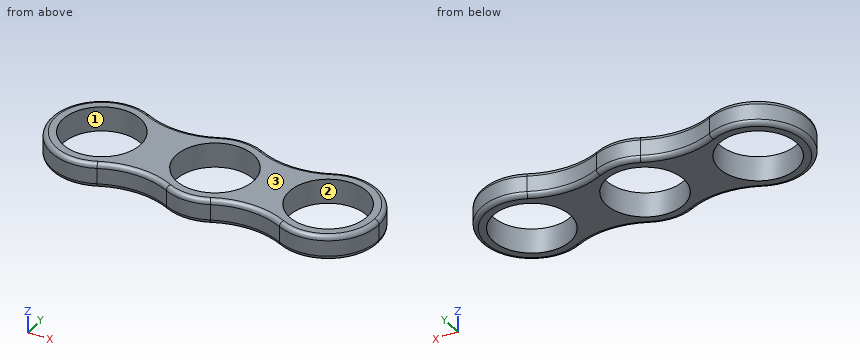
```python
from build123d import *

# Parameters (mm, degrees)
F0_R     = 11
F1_DEPTH = 7
F2_R     = 1.27


with BuildPart() as f1:
    # F0 (on Top) → F1 (new body)
    with BuildSketch(Plane.XY):
        with BuildLine():
            ThreePointArc((6.1706337368, -12.8862692637), (12.0891601396, -7.6147792724), (14.2875, 0))
            ThreePointArc((14.2875, 0), (12.0891601396, 7.6147792724), (6.1706337368, 12.8862692637))
            ThreePointArc((6.1706337368, 12.8862692637), (0, 14.2875), (-6.1706337368, 12.8862692637))
            ThreePointArc((-6.1706337368, 12.8862692637), (-14.2875, 0), (-6.1706337368, -12.8862692637))
            ThreePointArc((-6.1706337368, -12.8862692637), (0, -14.2875), (6.1706337368, -12.8862692637))
        make_face()
        Circle(F0_R, mode=Mode.SUBTRACT)
        with BuildLine():
            ThreePointArc((6.1706337368, 12.8862692637), (12.0891601396, 7.6147792724), (14.2875, 0))
            ThreePointArc((14.2875, 0), (12.0891601396, -7.6147792724), (6.1706337368, -12.8862692637))
            ThreePointArc((6.1706337368, -12.8862692637), (15.875, -10.6825966971), (25.5793662632, -12.8862692637))
            ThreePointArc((25.5793662632, -12.8862692637), (17.4625, 0), (25.5793662632, 12.8862692637))
            ThreePointArc((25.5793662632, 12.8862692637), (15.875, 10.6825966971), (6.1706337368, 12.8862692637))
        make_face()
        with BuildLine():
            ThreePointArc((-6.1706337368, -12.8862692637), (-14.2875, 0), (-6.1706337368, 12.8862692637))
            ThreePointArc((-6.1706337368, 12.8862692637), (-15.875, 10.6825966971), (-25.5793662632, 12.8862692637))
            ThreePointArc((-25.5793662632, 12.8862692637), (-19.6608398604, 7.6147792724), (-17.4625, 0))
            ThreePointArc((-17.4625, 0), (-19.6608398604, -7.6147792724), (-25.5793662632, -12.8862692637))
            ThreePointArc((-25.5793662632, -12.8862692637), (-15.875, -10.6825966971), (-6.1706337368, -12.8862692637))
        make_face()
        with BuildLine():
            ThreePointArc((46.0375, 0), (39.3647792724, 12.0891601396), (25.5793662632, 12.8862692637))
            ThreePointArc((25.5793662632, 12.8862692637), (17.4625, 0), (25.5793662632, -12.8862692637))
            ThreePointArc((25.5793662632, -12.8862692637), (39.3647792724, -12.0891601396), (46.0375, 0))
        make_face()
        with Locations((31.75, 0)):
            Circle(F0_R, mode=Mode.SUBTRACT)
        with BuildLine():
            ThreePointArc((-17.4625, 0), (-19.6608398604, 7.6147792724), (-25.5793662632, 12.8862692637))
            ThreePointArc((-25.5793662632, 12.8862692637), (-46.0375, 0), (-25.5793662632, -12.8862692637))
            ThreePointArc((-25.5793662632, -12.8862692637), (-19.6608398604, -7.6147792724), (-17.4625, 0))
        make_face()
        with Locations((-31.75, 0)):
            Circle(F0_R, mode=Mode.SUBTRACT)
    extrude(amount=F1_DEPTH)

    # F2
    f2_edges = [f1.edges().sort_by_distance(p)[0] for p in [
        (-46.0375, 0, 7),
        (0, 14.2875, 0),
    ]]
    fillet(f2_edges, radius=F2_R)


solid = f1.part
```
Work out the finished part from the listing and answer in its coordinate system (mm). Face numbers are marked on the shaded views. Coordinates: 2 decimals unless noted, no trailing zeros. Loops run counter-clockwise (first coordinate to the right, second up) from the corner with the lowest first, then second, coordinate; pieces in that order, holes last.
1) Flat-ended cylindrical pins translate along their axes: pin 1 (1 mm diameter, centred on x = -35.5, z = 2.5, fed in from -Y); pin 2 (1 mm diameter, centred on x = -28, z = 2.5, fed in from +Y); pin 3 (2 mm diameter, centred on y = 3.5, z = 3, fed in from +X). Find the tip coordinate at first contact, or state that the pin passes through.
Results:
pin 1: stops at y = -13.91
pin 2: stops at y = 13.91
pin 3: stops at x = 45.82
2) Consider probe 1 along Y at (x, z) = (31.75, 3); probe 2 along X at (y, z) = (-8.5, 3.5); probe 3 along X at (y, z) = (-3, 1). Determine where each line is inside the solid, lowest interval first.
Results:
probe 1: y = -14.29 to -11, 11 to 14.29
probe 2: x = -43.23 to -38.73, -24.77 to -6.98, 6.98 to 24.77, 38.73 to 43.23
probe 3: x = -45.69 to -42.33, -21.17 to -10.58, 10.58 to 21.17, 42.33 to 45.69
3) Section B-B (z = 3.5) is taken. Give the number of separate pieces and of enclosed holes in the cut face, plus the area to 3 significant figures.
Results:
separate pieces: 1
enclosed holes: 3
area: 1,070 mm2
4) For a pull along X with two mould halves and no side action, classify the marked faces 1, 2 and 3 as +X half, -X half, draft (parallel to the pull), parting line (faces both ways), or undercut.
Results:
face 1: undercut
face 2: undercut
face 3: draft
5) Section A-A (x = 0) is taken. Give the vertices of the cut face in (y, z).
Results:
outline: (-14.29, 1.27) arc R1.27 ccw to (-13.02, 0) - (-11, 0) - (-11, 7) - (-13.02, 7) arc R1.27 ccw to (-14.29, 5.73) - close; (11, 0) - (13.02, 0) arc R1.27 ccw to (14.29, 1.27) - (14.29, 5.73) arc R1.27 ccw to (13.02, 7) - (11, 7) - close
